Print and shaded views of the part. All mm, measured from the part's lowest x, y and z. A direction names the side the tool comes from. Coordinates: 2 decimals unless noted, no trailing zeros. Order: outer loops, then holes, each group sorted by start corner. A loop starts at its lowest first (then second) coordinate and runs counter-clockwise, first axis right, second up. Notation, with made-up numbers: (47, 69.5) - (86, 69.5) arc R13 cw to (86, 74.5) - close; hole circle Ø10 at (33.5, 43.5). An arc over 180 degrees is marked (long way). Write each question's results on one line, items separated by ' | '.
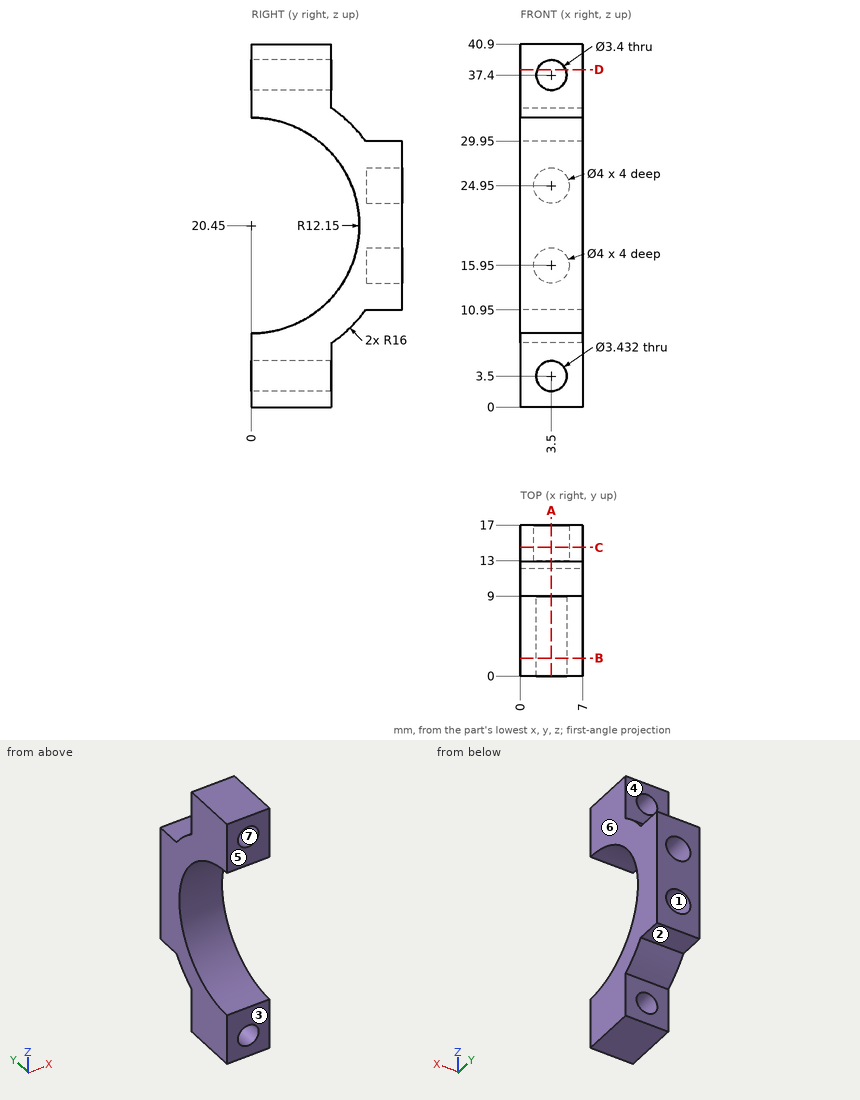
1. Band-saw the part on B-B on y = 2. Give the cut face in (x, z) (1 decimal), then the cut area to 3 significant figures.
Solved:
outline: (0, 0) - (7, 0) - (7, 8.5) - (0, 8.5) - close; (0, 32.4) - (7, 32.4) - (7, 40.9) - (0, 40.9) - close; hole circle Ø3.4 at (3.5, 3.5); hole circle Ø3.4 at (3.5, 37.4) | area: 100 mm2
2. Drop flat-ended pins along their axis: pin 1 Ø4 at (x, z) = (3, 27) entering from -Y; pin 2 Ø1.2 at (x, y) = (4, 14.5) entering from -Z; pin 3 Ø1.2 at (x, y) = (5, 14.5) entering from +Z. Give the stop position or say it passes through.
Solved:
pin 1: stops at y = 8.63 | pin 2: stops at z = 10.95 | pin 3: stops at z = 29.95
3. Band-saw the part on C-C on y = 14.5. Give the cut face in (x, z).
Solved:
outline: (0, 10.95) - (7, 10.95) - (7, 29.95) - (0, 29.95) - close; hole circle Ø4 at (3.5, 15.95); hole circle Ø4 at (3.5, 24.95)
4. Band-saw the part on A-A on x = 3.5. Give the number of separate pieces and of enclosed holes in the cut face, then the cut area to 3 significant figures.
Solved:
separate pieces: 3 | enclosed holes: 0 | area: 211 mm2
5. Tool access for the marked faces 1, 2, 3 and 4: list every direction of +Z, -Z, +X, -X, +Y, -Y with a clear straight run to the whole face (end or side of a thin tool).
Solved:
face 1: +Y | face 2: -Z, +X, -X, +Y | face 3: +Z, -Z, +X, -X, -Y | face 4: +Z, +X, -X, +Y
6. Probe line 1 (Z direction, x = 3.5, y = 14); line 2 (X direction, y = 3.5, z = 37.4); line 3 (X direction, y = 14.85, z = 15.95). List the from-to ranges inside material, lowest first.
Solved:
line 1: z = 10.95 to 13.95, 17.95 to 22.95, 26.95 to 29.95 | line 2: x = 0 to 1.8, 5.2 to 7 | line 3: x = 0 to 1.5, 5.5 to 7
7. Two-plate mould, pull along X, no slides. Class the marked faces 5, 6 and 7: +X half, -X half, draft (parallel to the pull), parting line (faces both ways), or undercut.
Solved:
face 5: draft | face 6: +X half | face 7: undercut
8. Band-saw the part on D-D on z = 38. Give the cut face in (x, y).
Solved:
outline: (0, 0) - (1.91, 0) - (1.91, 9) - (0, 9) - close; (5.09, 0) - (7, 0) - (7, 9) - (5.09, 9) - close
